The listing builds one solid part. Answer for the finished solid, in the listing's coordinates (mm). A direction names the side the tool comes from. Round coordinates to 2 decimals unless told otherwise and drop trailing zeros. Write each loop counter-clockwise with the first axis right and the second up, starting at its lowest first coordinate (ties: lowest second). Pieces come first, ordered by that corner, then holes. Notation, with made-up numbers: M 75,-39 L 81,-39 A30 ccw 81,-14 Z; hole C 46.5,29.25 d5. An arc over 180 degrees is marked long. Write each question's results on one line, items separated by ' | '.
from build123d import *
from build123d.topology import SkipClean

# Parameters (mm, degrees)
ESQUISSE1_R             = 1.4
ESQUISSE1_R_2           = 0.75
BOSS_EXTRU_1_DEPTH      = 2
ESQUISSE2_R             = 3.9
ESQUISSE2_R_2           = 3
BOSS_EXTRU_2_DEPTH      = 0.5
ENL_V_START             = -1.2
ESQUISSE3_R             = 3
ENL_V_MAT_EXTRU_1_DEPTH = 1.2
BOSS_EXTRU_3_START      = 2.5
ESQUISSE4_R             = 4.5
ESQUISSE4_R_2           = 2.75
BOSS_EXTRU_3_DEPTH      = 2.5


with BuildPart() as part:
    # Esquisse1 → Boss.-Extru.1 (new body)
    with BuildSketch(Plane.XY):
        with BuildLine():
            Line((-0.620689655, 4.45698826), (-14.844827586, 2.476104589))
            ThreePointArc((-14.844827586, 2.476104589), (-17, 0), (-14.844827586, -2.476104589))
            Line((-14.844827586, -2.476104589), (-0.620689655, -4.45698826))
            ThreePointArc((-0.620689655, -4.45698826), (0, -4.5), (0.620689655, -4.45698826))
            Line((0.620689655, -4.45698826), (14.844827586, -2.476104589))
            ThreePointArc((14.844827586, -2.476104589), (17, 0), (14.844827586, 2.476104589))
            Line((14.844827586, 2.476104589), (0.620689655, 4.45698826))
            ThreePointArc((0.620689655, 4.45698826), (0, 4.5), (-0.620689655, 4.45698826))
        make_face()
        Circle(ESQUISSE1_R, mode=Mode.SUBTRACT)
        with Locations((14.5, 0)):
            Circle(ESQUISSE1_R_2, mode=Mode.SUBTRACT)
        with Locations((-14.5, 0)):
            Circle(ESQUISSE1_R_2, mode=Mode.SUBTRACT)
        with Locations((-12, 0)):
            Circle(ESQUISSE1_R_2, mode=Mode.SUBTRACT)
        with Locations((-9.5, 0)):
            Circle(ESQUISSE1_R_2, mode=Mode.SUBTRACT)
        with Locations((9.5, 0)):
            Circle(ESQUISSE1_R_2, mode=Mode.SUBTRACT)
        with Locations((12, 0)):
            Circle(ESQUISSE1_R_2, mode=Mode.SUBTRACT)
    extrude(amount=BOSS_EXTRU_1_DEPTH)

    # Esquisse2 → Boss.-Extru.2 (add)
    with BuildSketch(Plane.XY.offset(2)):
        with Locations(Location((0, 0, 0), (0, 0, 180))):
            Circle(ESQUISSE2_R)
        Circle(ESQUISSE2_R_2, mode=Mode.SUBTRACT)
    extrude(amount=BOSS_EXTRU_2_DEPTH)

    # Esquisse3 → Enlèv. mat.-Extru.1 (cut)
    with BuildSketch(Plane.XY.offset(2.5).offset(ENL_V_START)):
        Circle(ESQUISSE3_R)
    extrude(amount=ENL_V_MAT_EXTRU_1_DEPTH, mode=Mode.SUBTRACT)

    # Esquisse4 → Boss.-Extru.3 (add)
    with SkipClean():  # the faces are left unmerged after this step: merging them gives an invalid solid
        with BuildSketch(Plane(origin=(0, 0, 0), x_dir=(-1, 0, 0), z_dir=(0, 0, -1)).offset(BOSS_EXTRU_3_START)):
            Circle(ESQUISSE4_R)
            Circle(ESQUISSE4_R_2, mode=Mode.SUBTRACT)
        extrude(amount=-BOSS_EXTRU_3_DEPTH)


solid = part.part
1) Section D-D (z = -1.5) is taken. Determine the outline of the cut face in (x, y).
Return value:
outline: C 0,0 d9; hole C 0,0 d5.5
2) Find the intervals of material crossed by line 1 (Y direction, x = 0, z = 0.4); line 2 (Z direction, x = 4.5, y = 3); line 3 (Y direction, x = -0.5, z = -0.2), in increasing order.
Return value:
line 1: -4.5 to -1.4, 1.4 to 4.5 | line 2: 0 to 2 | line 3: -4.47 to -2.7, 2.7 to 4.47
3) A tool of negligible diameter and unlimited length cuts with its end or side. For faces 5 (the face through (-15.25, 0.03, 0.99)), 6 (the face through (1.2, -1.2, 0)), from which of +Z, -Z, +X, -X, +Y, -Y can it reach the whole face along a straight path? Write none if from no direction.
Return value:
face 5: +Z, -Z | face 6: -Z
4) Section B-B (y = 2) is taken. Determine the outline of the cut face in (x, z).
Return value:
outline: M -16,0 L -4.03,0 L -4.03,-2.5 L -1.89,-2.5 L -1.89,0 L 1.89,0 L 1.89,-2.5 L 4.03,-2.5 L 4.03,0 L 16,0 L 16,2 L 3.35,2 L 3.35,2.5 L 2.24,2.5 L 2.24,1.3 L -2.24,1.3 L -2.24,2.5 L -3.35,2.5 L -3.35,2 L -16,2 Z
5) Each of these flat-tipped pins is pushed along its axis until it touches: pin 1 (4.5 mm diameter, centred on x = 13, y = 0.5, fed in from -Z); pin 2 (1.4 mm diameter, centred on x = -9.5, y = 0, fed in from +Z); pin 3 (3 mm diameter, centred on x = -10.5, z = -1, fed in from -Y); pin 4 (2 mm diameter, centred on x = 8, y = 1.5, fed in from +Z). Where does it stop, or does it pass through?
Return value:
pin 1: z = 0 | pin 2: through | pin 3: y = -3.24 | pin 4: z = 2
6) The mould has two halves that part along Y. Classify faces 1 (the face through (0, -3, -2.5)), 2 (the face through (17, 0, 1)), 3 (the face through (-3, 0, 2)), 4 (the face through (-7.832, -3.453, 0.986)): +Y half, -Y half, draft (parallel to the pull), parting line (faces both ways), or undercut.
Return value:
face 1: draft | face 2: parting line | face 3: undercut | face 4: -Y half
7) Section C-C (x = -2) is taken. Determine the outline of the cut face in (y, z), then the cut area to 3 significant figures.
Return value:
outline: M -4.26,0 L -4.03,0 L -4.03,-2.5 L -1.89,-2.5 L -1.89,0 L 1.89,0 L 1.89,-2.5 L 4.03,-2.5 L 4.03,0 L 4.26,0 L 4.26,2 L 3.35,2 L 3.35,2.5 L 2.24,2.5 L 2.24,1.3 L -2.24,1.3 L -2.24,2.5 L -3.35,2.5 L -3.35,2 L -4.26,2 Z | area: 25.8 mm²
8) Section A-A (x = -14.5) is taken. Determine the outline of the cut face in (y, z), then the cut area to 3 significant figures.
Return value:
outline: M -2.52,0 L -0.75,0 L -0.75,2 L -2.52,2 Z; M 0.75,0 L 2.52,0 L 2.52,2 L 0.75,2 Z | area: 7.10 mm²
